Autodesk Inventor part; units mm, degrees
ref_plane "YZ Plane" through (0, 0, 0) normal (1, 0, 0) x (0, 1, 0)
ref_plane "XZ Plane" through (0, 0, 0) normal (0, 1, 0) x (-1, 0, 0)
ref_plane "XY Plane" through (0, 0, 0) normal (0, 0, 1) x (1, 0, 0)
sketch "Sketch1" plane through (0, 0, 0) normal (0, 0, 1) x (1, 0, 0)
  line L0 (0, 0) -> (-26.7469, 1.7445) construction
  line L1 (-26.7469, 1.7445) -> (0, 27.7395) construction
  line L2 (0, 27.7395) -> (0, 0) construction
  line L3 (-0.2603, -3.9915) -> (-27.0072, -2.247)
  line L4 (-29.5347, 4.6129) -> (-2.7878, 30.6079)
  line L5 (4, 27.7395) -> (4, 0)
  arc A0 (4, 27.7395) -> (-2.7878, 30.6079) centre (0, 27.7395) ccw
  arc A1 (-29.5347, 4.6129) -> (-27.0072, -2.247) centre (-26.7469, 1.7445) ccw
  arc A2 (-0.2603, -3.9915) -> (4, 0) centre (0, 0) ccw
  dimension "d6" = 37.2979
  dimension "d14" = 27.7395
  dimension "d15" = 26.8037
  dimension "d18" = 4
extrude "Extrusion1" add sketch "Sketch1" along normal mid plane 20
sketch "Sketch2" plane through (0, 0, 0) normal (0, 0, 1) x (1, 0, 0)
  arc A0 (4, 27.7395) -> (-2.7878, 30.6079) centre (0, 27.7395) ccw
  line L0 (-29.5347, 4.6129) -> (-25.7337, 8.3071)
  arc A1 (-29.5347, 4.6129) -> (-27.0072, -2.247) centre (-26.7469, 1.7445) ccw
  line L1 (-0.2603, -3.9915) -> (-10.9499, -3.2943)
  arc A2 (-0.2603, -3.9915) -> (4, 0) centre (0, 0) ccw
  line L2 (4, 27.7395) -> (4, 10.5666)
  line L3 (-25.7337, 8.3071) -> (-13.5738, -3.1232)
  line L4 (-25.7337, 8.3071) -> (-5.6497, 27.8265) construction
  line L5 (-13.5738, -3.1232) -> (-27.0072, -2.247)
  line L6 (-5.6497, 27.8265) -> (4, 10.5666)
  line L7 (4, 9.0015) -> (-10.9499, -3.2943)
  line L8 (4, 10.5666) -> (4, 9.0015) construction
  line L9 (4, 9.0015) -> (4, 0)
  line L10 (-10.9499, -3.2943) -> (-13.5738, -3.1232) construction
  line L11 (-5.6497, 27.8265) -> (-2.7878, 30.6079)
  arc A3 (-0.2603, -3.9915) -> (4, 0) centre (0, 0) ccw
  point P0 (0, 0)
extrude "Extrusion2" cut sketch "Sketch2" along normal mid plane 10
sketch "Sketch3" plane through (0, 0, 10) normal (0, 0, 1) x (1, 0, 0)
  arc A0 (4, 27.7395) -> (-2.7878, 30.6079) centre (0, 27.7395) ccw construction
  arc A1 (-29.5347, 4.6129) -> (-27.0072, -2.247) centre (-26.7469, 1.7445) ccw construction
  arc A2 (-0.2603, -3.9915) -> (4, 0) centre (0, 0) ccw construction
hole "Hole1" at (-26.7469, 1.7445, 10) at (0, 0, 10) at (0, 27.7395, 10) direction (0, 0, -1) diameter 3.4 end through all
fillet "Fillet1" radius 2 6 edges at (-13.5738, -3.1232, 0) (-10.9499, -3.2943, 0) (-25.7337, 8.3071, 0) (-5.6497, 27.8265, 0) (4, 10.5666, 0) (4, 9.0015, 0)
equation "\"d6\" = LengthE"
equation "\"d14\" = LengthB"
equation "\"d15\" = LengthD"
equation "\"ScaleFactor\" = 1"
equation "\"LengthA\" = 2.54 * ScaleFactor"
equation "\"LengthB\" = 2.77395 * ScaleFactor"
equation "\"LengthC\" = 2.6269 * ScaleFactor"
equation "\"LengthD\" = 2.68037 * ScaleFactor"
equation "\"LengthE\" = 3.72979 * ScaleFactor"
equation "\"LengthF\" = 2.63358 * ScaleFactor"
equation "\"LengthG\" = 2.4531 * ScaleFactor"
equation "\"LengthH\" = 4.39153 * ScaleFactor"
equation "\"LengthI\" = 3.27525 * ScaleFactor"
equation "\"LengthJ\" = 3.3421 * ScaleFactor"
equation "\"LengthK\" = 3.81 * ScaleFactor"
equation "\"LengthL\" = 0.521368 * ScaleFactor"
equation "\"LengthM\" = 1.00263 * ScaleFactor"
equation "\"d0\" = LengthA"
equation "\"d1\" = LengthJ"
equation "\"d2\" = LengthM"
equation "\"d3\" = LengthL"
equation "\"d4\" = LengthB"
equation "\"d5\" = LengthC"
equation "\"d7\" = LengthD"
equation "\"d8\" = LengthE"
equation "\"d9\" = LengthF"
equation "\"d10\" = LengthG"
equation "\"d11\" = LengthH"
equation "\"d12\" = LengthI"
equation "\"d13\" = LengthK"
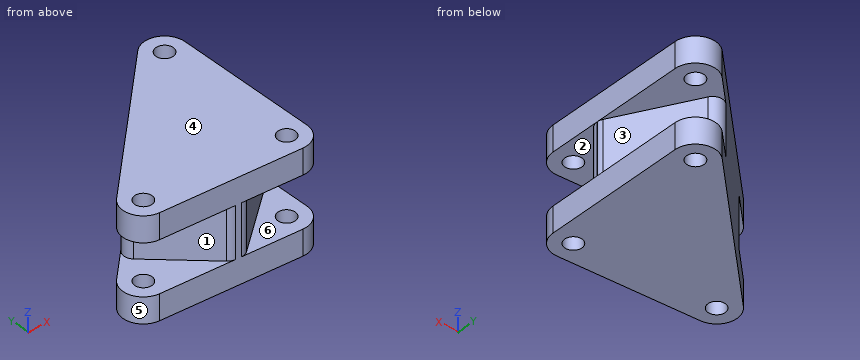
The model under review builds one solid part; all positions refer to its coordinate system, in mm. Face numbers are marked on the shaded views. A direction names the side the tool comes from. Round coordinates to 2 decimals unless told otherwise and drop trailing zeros. Loops run counter-clockwise (first coordinate to the right, second up) from the corner with the lowest first, then second, coordinate; pieces in that order, holes last.
1) Consider section A-A on z = 6.75. State the section outline as (x, y) points.
Values follow:
outline: (-29.53, 4.61) arc R4 ccw to (-27.01, -2.25) - (-0.26, -3.99) arc R4 ccw to (4, 0) - (4, 27.74) arc R4 ccw to (-2.79, 30.61) - close; hole circle Ø3.4 at (-26.75, 1.74); hole circle Ø3.4 at (0, 0); hole circle Ø3.4 at (0, 27.74)
2) Tool access review of the marked faces 1, 2 and 3: name each direction out of +Z, -Z, +X, -X, +Y, -Y from which nothing blocks a thin tool from reaching the whole face with its end or side.
Values follow:
face 1: -X, -Y
face 2: +X, -Y
face 3: +X, +Y
3) The part is to be moulded in two halves that separate along Z. For the marked faces 4, 5 and 6, say which applies: pulls with the +Z half, pulls with the -Z half, needs draft (parallel to the pull), parting line crosses it, or undercut.
Values follow:
face 4: pulls with the +Z half
face 5: needs draft
face 6: undercut
4) Wall thickness on line 1 along Y through (x, z) = (0, 6.75); line 2 along Z through (x, y) = (-1, 29.5); line 3 along X through (y, z) = (0, -7.25): over which ranges is each line inside the solid? List them lowest first.
Values follow:
line 1: y = -4 to -1.7, 1.7 to 26.04, 29.44 to 31.74
line 2: z = -10 to -5, 5 to 10
line 3: x = -30.35 to -1.7, 1.7 to 4
5) Consider section D-D on y = 10.5. State the section outline as (x, z) points, then the cut area to 3 significant figures.
Values follow:
outline: (-23.48, -10) - (4, -10) - (4, -5) - (3.95, -5) - (3.95, 5) - (4, 5) - (4, 10) - (-23.48, 10) - close
area: 549 mm2
6) Consider section C-C on x = -19. State the section outline as (y, z) points, then the cut area to 3 significant figures.
Values follow:
outline: (-2.77, -10) - (14.85, -10) - (14.85, 10) - (-2.77, 10) - (-2.77, 5) - (1.98, 5) - (1.98, -5) - (-2.77, -5) - close
area: 305 mm2
7) Clearance check with flat-ended pins moving along their axes: P1, Ø3, axis at y = 0, z = -2.5, coming from the -X side; P2, Ø10, axis at x = -16, z = -7, coming from the -Y side; P3, Ø10, axis at x = -24, z = -3, coming from the -Y side. State where each tip first meets the part, or that it passes through.
Values follow:
P1: stops at x = -18.49
P2: stops at y = -3.29
P3: stops at y = -2.74
8) Consider section B-B on y = 1. State the section outline as (x, z) points.
Values follow:
outline: (-30.68, -10) - (-28.28, -10) - (-28.28, -5) - (-30.68, -5) - close; (-30.68, 5) - (-28.28, 5) - (-28.28, 10) - (-30.68, 10) - close; (-25.22, -10) - (-1.37, -10) - (-1.37, -5) - (-5.73, -5) - (-5.73, 5) - (-1.37, 5) - (-1.37, 10) - (-25.22, 10) - (-25.22, 5) - (-17.96, 5) - (-17.96, -5) - (-25.22, -5) - close; (1.37, -10) - (4, -10) - (4, -5) - (1.37, -5) - close; (1.37, 5) - (4, 5) - (4, 10) - (1.37, 10) - close
